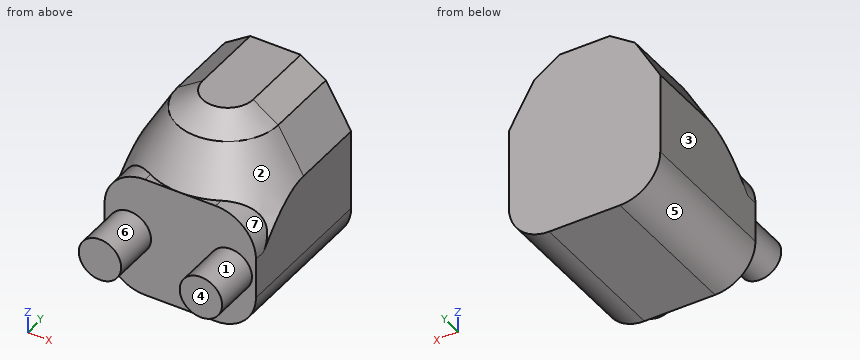
from build123d import *

# Parameters (mm, degrees)
F0_W     = 19.05
F0_H     = 15.24
F1_DEPTH = 9.525
F2_R     = 2.667
F3_DEPTH = 5.969
F8_R     = 5.08


with BuildPart() as f1:
    # F0 (on Right) → F1 (new body, symmetric)
    with BuildSketch(Plane.YZ):
        with Locations((-9.525, 7.62)):
            Rectangle(F0_W, F0_H)
    extrude(amount=F1_DEPTH, both=True)

    # F2 (on face) → F3 (join)
    with BuildSketch(Plane.XZ.offset(19.05)):
        with Locations((6.35, 7.62)):
            Circle(F2_R)
        with Locations((-6.35, 7.62)):
            Circle(F2_R)
    extrude(amount=F3_DEPTH)

    # F4 (on Right) → F5 (revolve)
    with BuildSketch(Plane.YZ):
        Polygon((-19.05, 15.24), (-9.525, 15.24), (-9.525, 22.86), (-12.7, 22.86), (-15.875, 20.739261314), align=None)
    revolve(axis=Axis((0, -9.525, 19.05), (0, 0, 1)))

    # F6 (on face) → F7 (join, up to the next surface of F1)
    with BuildSketch(Plane(origin=(0, 0, 0), x_dir=(-1, 0, 0), z_dir=(0, 1, 0))):
        Polygon((-6.35, 20.739261314), (-9.525, 15.24), (0, 15.24), (9.525, 15.24), (6.35, 20.739261314), (3.175, 22.86), (-3.175, 22.86), align=None)
    extrude(until=Until.NEXT, dir=(0, -1, 0))

    # F8
    f8_edges = [f1.edges().sort_by_distance(p)[0] for p in [
        (9.525, -14.2875, 15.24),
        (-9.525, -14.2875, 15.24),
        (-9.525, -9.525, 0),
        (9.525, -9.525, 0),
    ]]
    fillet(f8_edges, radius=F8_R)


solid = f1.part
Geometry: final body of the model. Coordinates: model frame, mm. Face numbers are marked on the shaded views. A direction names the side the tool comes from. Coordinates: 2 decimals unless noted, no trailing zeros. Order: outer loops, then holes, each group sorted by start corner. A loop starts at its lowest first (then second) coordinate and runs counter-clockwise, first axis right, second up.
(1) Draft query along X for the marked faces 1, 2, 3 and 4. Return one class per face: pulls with the +X half, pulls with the -X half, needs draft (parallel to the pull), parting line crosses it, or undercut.
(2) Material intervals for probe 1 along Y at (x, z) = (-1, 15); probe 2 along Z at (x, y) = (-4, -18.25); probe 3 along X at (y, z) = (-6.75, 2), sorted ascending.
(3) Section query C-C (y = -21). Return the cut outline in (x, z), plus the area to 3 significant figures.
(4) First-contact query: pin 1 (0.6 mm diameter, centred on x = -1.5, y = -18.5, fed in from +Z); pin 2 (0.6 mm diameter, centred on x = 2.5, y = -18.5, fed in from +Z); pin 3 (10 mm diameter, centred on x = 5.5, z = 18, fed in from -Y); pin 4 (3 mm diameter, centred on y = -21, z = 17, fed in from -X). Flat tips, straight axial feed; report the tip coordinate or a pass-through.
(5) Section query D-D (z = 13). Return the cut outline in (x, y) (3 decimals), plus the area to 3 significant figures.
(6) Section query A-A (z = 7.62). Return the cut outline in (x, y) (3 decimals).
(7) Access query for the marked faces 5, 6 and 7. Directions: +Z, -Z, +X, -X, +Y, -Y. A direction counts if a zero-diameter tool reaches every point of the face in a straight line with its end or side. Return the directions, or none.
(8) Section query B-B (y = -4.5). Return the cut outline in (x, z) (3 decimals).
Solution:
1. face 1: undercut
1. face 2: parting line crosses it
1. face 3: pulls with the -X half
1. face 4: needs draft
2. probe 1: y = -19.05 to 0
2. probe 2: z = 0 to 15.24
2. probe 3: x = -8.48 to 8.48
3. outline: circle Ø5.33 at (-6.35, 7.62); circle Ø5.33 at (6.35, 7.62)
3. area: 44.7 mm2
4. pin 1: stops at z = 16.5
4. pin 2: stops at z = 16.12
4. pin 3: stops at y = -19.05
4. pin 4: passes through
5. outline: (-9.525, -14.654) arc R10.818 ccw to (-8.657, -16.013) - (-8.657, -19.05) - (8.657, -19.05) - (8.657, -16.013) arc R10.818 ccw to (9.525, -14.654) - (9.525, 0) - (-9.525, 0) - close
5. area: 357 mm2
6. outline: (-9.525, -19.05) - (-9.017, -19.05) - (-9.017, -25.019) - (-3.683, -25.019) - (-3.683, -19.05) - (3.683, -19.05) - (3.683, -25.019) - (9.017, -25.019) - (9.017, -19.05) - (9.525, -19.05) - (9.525, 0) - (-9.525, 0) - close
7. face 5: -Z, -X, +Y, -Y
7. face 6: -Y
7. face 7: +Z, +X, -Y
8. outline: (-9.525, 5.08) arc R5.08 ccw to (-4.445, 0) - (4.445, 0) arc R5.08 ccw to (9.525, 5.08) - (9.525, 15.24) - (6.35, 20.739) - (3.175, 22.86) - (-3.175, 22.86) - (-6.35, 20.739) - (-9.525, 15.24) - close
